The listing builds one solid part. Answer for the finished solid, in the listing's coordinates (mm). Face numbers are marked on the shaded views. A direction names the side the tool comes from. Give positions to 0.01 mm unless a question says otherwise; leave off trailing zeros. Loops run counter-clockwise (first coordinate to the right, second up) from the corner with the lowest first, then second, coordinate; pieces in that order, holes last. Notation, with made-up numbers: (11.5, 71) - (48.5, 71) arc R34 cw to (48.5, 102) - close; hole circle Ø8 at (42, 32). An arc over 180 degrees is marked (long way). Write item = value, one per line. Start each with the question number.
1) Flat-ended cylindrical pins translate along their axes: P1, Ø1.5, axis at x = 12.5, z = 8, coming from the +Y side; P2, Ø5.5, axis at x = 4, y = -10, coming from the +Z side. Find the tip coordinate at first contact, or state that the pin passes through.
2) The part is cut by section C-C on z = 40.5. Write down the section's boundary in (x, y).
3) Which of the six approach directions +Z, -Z, +X, -X, +Y, -Y give full straight-line access (tool end or side, diameter ignored) to the marked faces 4, 5 and 6?
4) The mould has two halves that part along X. Classify the marked faces 1, 2 and 3: +X half, -X half, draft (parallel to the pull), parting line (faces both ways), or undercut.
5) The part is cut by section B-B on x = 20. Write down the section's boundary in (y, z), plus the area to 3 significant figures.
6) The part is cut by section A-A on z = -1. Write down the section's boundary in (x, y), plus the area to 3 significant figures.
7) Consider probe 1 along X at (y, z) = (-13, 20.5); probe 2 along X at (y, z) = (-2, -6.5); probe 3 along Z at (x, y) = (73.5, -11.25). Determine where each line is inside the solid, lowest interval first.
8) The part is cut by section D-D on y = -10.75. Write down the section's boundary in (x, z), plus the area to 3 significant figures.
from build123d import *

# Parameters (mm, degrees)
F1_DEPTH     = 20
F2_F1_R      = 1
F2_F2_R      = 1
F3_T1_DEPTH  = 63
F3_T3_DEPTH  = 28
F3_T5_DEPTH  = 167
F3_T7_DEPTH  = 78
F3_S11_W     = 1
F3_S11_H     = 1
F3_T12_DEPTH = 1
F3_S17_W     = 1
F3_S17_H     = 1
F3_T18_DEPTH = 1
F3_T22_ANGLE = 90
F3_T24_ANGLE = 90
F3_T26_ANGLE = 90


# Not quite as in the source:
# - a fillet or chamfer that OpenCascade refuses, or shapes differently, is made with other operations: its cross-section is extruded or revolved along the edge and cut away or added


with BuildPart() as f1:
    # F0 (on Front) → F1 (new body)
    with BuildSketch(Plane.XZ):
        Polygon((-54.7987632453, 48.7000103295), (-54.7987632453, -31.2999896705), (114.2012367547, -31.2999896705), (114.2012367547, 33.7000103295), (84.2012367547, 33.7000103295), (84.2012367547, -11.2999896705), (42.2012367547, -11.2999896705), (42.2012367547, 8.7000103295), (-24.7987632453, 8.7000103295), (-24.7987632453, 48.7000103295), align=None)
    extrude(amount=F1_DEPTH)

    # F2: fillet of radius 1 on 24 edges, made by hand

    # F2_f1
    f2_f1_edges = [f1.edges().sort_by_distance(p)[0] for p in [
        (-24.7987632453, -10, 8.7000103295),
        (84.2012367547, -10, -11.2999896705),
        (42.2012367547, -10, -11.2999896705),
    ]]
    fillet(f2_f1_edges, radius=F2_F1_R)

    # F2_f2
    f2_f2_edges = [f1.edges().sort_by_distance(p)[0] for p in [
        (-39.7987632453, -20, 48.7000103295),
        (9.2012367547, -20, 8.7000103295),
        (-24.7987632453, -20, 29.2000103295),
        (9.2012367547, 0, 8.7000103295),
        (-24.7987632453, -10, 48.7000103295),
        (42.2012367547, -10, 8.7000103295),
        (42.2012367547, -20, -0.7999896705),
        (63.2012367547, 0, -11.2999896705),
        (63.2012367547, -20, -11.2999896705),
        (114.2012367547, -10, 33.7000103295),
        (114.2012367547, 0, 1.2000103295),
        (99.2012367547, 0, 33.7000103295),
        (84.2012367547, 0, 11.7000103295),
        (-54.7987632453, 0, 8.7000103295),
        (29.7012367547, 0, -31.2999896705),
        (-54.7987632453, -10, -31.2999896705),
        (84.2012367547, -10, 33.7000103295),
        (-24.7987632453, 0, 29.2000103295),
        (-39.7987632453, 0, 48.7000103295),
        (114.2012367547, -10, -31.2999896705),
        (-54.7987632453, -10, 48.7000103295),
        (-24.5058700265, 0, 8.9929035483),
        (83.9083435358, 0, -11.0070964517),
        (83.9083435358, -20, -11.0070964517),
        (42.4941299735, -20, -11.0070964517),
        (42.4941299735, 0, -11.0070964517),
        (-24.5058700265, -20, 8.9929035483),
    ]]
    fillet(f2_f2_edges, radius=F2_F2_R)

    # F3: fillet of radius 1 on 7 edges, made by hand

    # F3_s2 → F3_t1 (cut)
    with BuildSketch(Plane.XY.offset(-30.2999896705)):
        with BuildLine():
            ThreePointArc((113.2012367547, -20), (113.9083435358, -19.7071067812), (114.2012367547, -19))
            Line((114.2012367547, -19), (114.2012367547, -20))
            Line((114.2012367547, -20), (113.2012367547, -20))
        make_face()
    extrude(amount=F3_T1_DEPTH, mode=Mode.SUBTRACT)

    # F3_s4 → F3_t3 (cut)
    with BuildSketch(Plane.YZ.offset(85.2012367547)):
        with BuildLine():
            ThreePointArc((-20, 32.7000103295), (-19.7071067812, 33.4071171107), (-19, 33.7000103295))
            Line((-19, 33.7000103295), (-20, 33.7000103295))
            Line((-20, 33.7000103295), (-20, 32.7000103295))
        make_face()
    extrude(amount=F3_T3_DEPTH, mode=Mode.SUBTRACT)

    # F3_s6 → F3_t5 (cut)
    with BuildSketch(Plane.YZ.offset(-53.7987632453)):
        with BuildLine():
            ThreePointArc((-20, -30.2999896705), (-19.7071067812, -31.0070964517), (-19, -31.2999896705))
            Line((-19, -31.2999896705), (-20, -31.2999896705))
            Line((-20, -31.2999896705), (-20, -30.2999896705))
        make_face()
    extrude(amount=F3_T5_DEPTH, mode=Mode.SUBTRACT)

    # F3_s8 → F3_t7 (cut)
    with BuildSketch(Plane.XY.offset(-30.2999896705)):
        with BuildLine():
            ThreePointArc((-53.7987632453, -20), (-54.5058700265, -19.7071067812), (-54.7987632453, -19))
            Line((-54.7987632453, -19), (-54.7987632453, -20))
            Line((-54.7987632453, -20), (-53.7987632453, -20))
        make_face()
    extrude(amount=F3_T7_DEPTH, mode=Mode.SUBTRACT)


with BuildPart() as f3_tool10:
    # F3_s11 → F3_t12 (new body)
    with BuildSketch(Plane.XZ.offset(19)):
        with Locations((-54.2987632453, 48.2000103295)):
            Rectangle(F3_S11_W, F3_S11_H)
    extrude(amount=F3_T12_DEPTH)

    # F3_s13 → F3_t14 (revolve, cut)
    with BuildSketch(Plane(origin=(-53.7987632453, -19, 47.7000103295), x_dir=(0.7071067812, 0, -0.7071067812), z_dir=(-0.7071067812, 0, -0.7071067812))):
        with BuildLine():
            ThreePointArc((0, -1), (1, 0), (0, 1))
            Line((0, 1), (0, -1))
        make_face()
    revolve(axis=Axis((-53.7987632453, -19, 47.7000103295), (0, -1, 0)), mode=Mode.SUBTRACT)


with BuildPart() as f1_1:
    add(f1.part)

    # F3_t9: cut F3_tool10
    add(f3_tool10.part, mode=Mode.SUBTRACT)


with BuildPart() as f3_tool16:
    # F3_s17 → F3_t18 (new body)
    with BuildSketch(Plane.XZ.offset(19)):
        with Locations((84.7012367547, 33.2000103295)):
            Rectangle(F3_S17_W, F3_S17_H)
    extrude(amount=F3_T18_DEPTH)

    # F3_s19 → F3_t20 (revolve, cut)
    with BuildSketch(Plane(origin=(85.2012367547, -19, 32.7000103295), x_dir=(0.7071067812, 0, -0.7071067812), z_dir=(-0.7071067812, 0, -0.7071067812))):
        with BuildLine():
            ThreePointArc((0, -1), (1, 0), (0, 1))
            Line((0, 1), (0, -1))
        make_face()
    revolve(axis=Axis((85.2012367547, -19, 32.7000103295), (0, -1, 0)), mode=Mode.SUBTRACT)


with BuildPart() as f1_2:
    add(f1_1.part)

    # F3_t15: cut F3_tool16
    add(f3_tool16.part, mode=Mode.SUBTRACT)

    # F3_s21 → F3_t22 (revolve, cut)
    with BuildSketch(Plane.YZ.offset(113.2012367547)):
        with BuildLine():
            ThreePointArc((-20, 32.7000103295), (-19.7071067812, 33.4071171107), (-19, 33.7000103295))
            Line((-19, 33.7000103295), (-20, 33.7000103295))
            Line((-20, 33.7000103295), (-20, 32.7000103295))
        make_face()
    revolve(axis=Axis((113.2012367547, -20, 32.7000103295), (0, 1, 0)), revolution_arc=F3_T22_ANGLE, mode=Mode.SUBTRACT)

    # F3_s23 → F3_t24 (revolve, cut)
    with BuildSketch(Plane.XY.offset(-30.2999896705)):
        with BuildLine():
            ThreePointArc((113.2012367547, -20), (113.9083435358, -19.7071067812), (114.2012367547, -19))
            Line((114.2012367547, -19), (114.2012367547, -20))
            Line((114.2012367547, -20), (113.2012367547, -20))
        make_face()
    revolve(axis=Axis((113.2012367547, -20, -30.2999896705), (0, 1, 0)), revolution_arc=F3_T24_ANGLE, mode=Mode.SUBTRACT)

    # F3_s25 → F3_t26 (revolve, cut)
    with BuildSketch(Plane.YZ.offset(-53.7987632453)):
        with BuildLine():
            ThreePointArc((-20, -30.2999896705), (-19.7071067812, -31.0070964517), (-19, -31.2999896705))
            Line((-19, -31.2999896705), (-20, -31.2999896705))
            Line((-20, -31.2999896705), (-20, -30.2999896705))
        make_face()
    revolve(axis=Axis((-53.7987632453, -20, -30.2999896705), (0, 1, 0)), revolution_arc=F3_T26_ANGLE, mode=Mode.SUBTRACT)


solid = f1_2.part
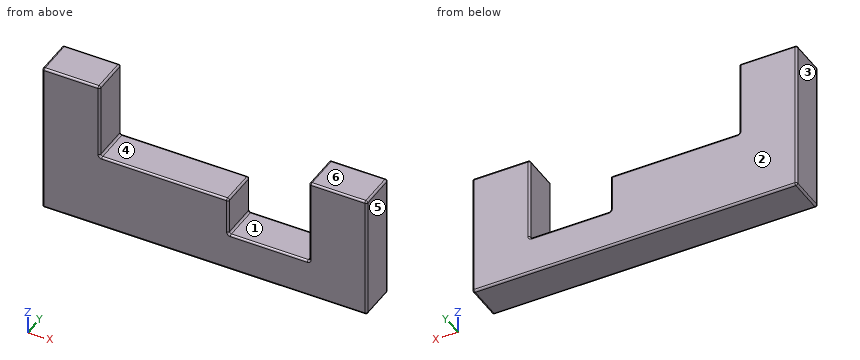
Answer below:
q1.P1 = 0
q1.P2 = 8.7
q2.outline = (-54.8, -19) arc R1 ccw to (-53.8, -20) - (-25.8, -20) arc R1 ccw to (-24.8, -19) - (-24.8, -1) arc R1 ccw to (-25.8, 0) - (-53.8, 0) arc R1 ccw to (-54.8, -1) - close
q3.face_4 = +Z, +Y, -Y
q3.face_5 = +Z, -Z, +X, +Y, -Y
q3.face_6 = +Z, +X, +Y, -Y
q4.face_1 = undercut
q4.face_2 = draft
q4.face_3 = -X half
q5.outline = (-20, -30.3) arc R1 ccw to (-19, -31.3) - (-1, -31.3) arc R1 ccw to (0, -30.3) - (0, 7.7) arc R1 ccw to (-1, 8.7) - (-19, 8.7) arc R1 ccw to (-20, 7.7) - close
q5.area = 799 mm2
q6.outline = (-54.8, -19) arc R1 ccw to (-53.8, -20) - (41.2, -20) arc R1 ccw to (42.2, -19) - (42.2, -1) arc R1 ccw to (41.2, 0) - (-53.8, 0) arc R1 ccw to (-54.8, -1) - close; (84.2, -19) arc R1 ccw to (85.2, -20) - (113.2, -20) arc R1 ccw to (114.2, -19) - (114.2, -1) arc R1 ccw to (113.2, 0) - (85.2, 0) arc R1 ccw to (84.2, -1) - close
q6.area = 2,540 mm2
q7.probe_1 = -54.8 to -24.8, 84.2 to 114.2
q7.probe_2 = -54.8 to 42.2, 84.2 to 114.2
q7.probe_3 = -31.3 to -11.3
q8.outline = (-54.8, -30.3) arc R1 ccw to (-53.8, -31.3) - (113.2, -31.3) arc R1 ccw to (114.2, -30.3) - (114.2, 32.7) arc R1 ccw to (113.2, 33.7) - (85.2, 33.7) arc R1 ccw to (84.2, 32.7) - (84.2, -10.3) arc R1 cw to (83.2, -11.3) - (43.2, -11.3) arc R1 cw to (42.2, -10.3) - (42.2, 7.7) arc R1 ccw to (41.2, 8.7) - (-23.8, 8.7) arc R1 cw to (-24.8, 9.7) - (-24.8, 47.7) arc R1 ccw to (-25.8, 48.7) - (-53.8, 48.7) arc R1 ccw to (-54.8, 47.7) - close
q8.area = 7,870 mm2
